from build123d import *

# Parameters (mm, degrees)
SKETCH_1_R          = 2.1
SKETCH_1_R_2        = 6.1
EXTRUDE_1_DEPTH     = 1.5
SKETCH_2_R          = 6.1
SKETCH_2_R_2        = 1.6
CUT_EXTRUDE_1_DEPTH = 53.758885508
FILLET_1_R          = 2


with BuildPart() as part:
    # ｽｹｯﾁ1 → ﾎﾞｽ - 押し出し1 (new body)
    with BuildSketch(Plane.XY):
        with BuildLine():
            ThreePointArc((-37.95979357, -17.309345429), (-38.658047176, -21.61823696), (-35, -24))
            Line((-35, -24), (-14.974979132, -24))
            ThreePointArc((-14.974979132, -24), (0, -35.5), (14.974979132, -24))
            Line((14.974979132, -24), (35, -24))
            ThreePointArc((35, -24), (38.658047176, -21.61823696), (37.95979357, -17.309345429))
            ThreePointArc((37.95979357, -17.309345429), (27.149823207, -3.034907568), (19.058822549, 12.938531129))
            ThreePointArc((19.058822549, 12.938531129), (17.587655142, 14.768604061), (15.342990138, 15.45779162))
            Line((15.342990138, 15.45779162), (-15.342990138, 15.45779162))
            ThreePointArc((-15.342990138, 15.45779162), (-17.587655142, 14.768604061), (-19.058822549, 12.938531129))
            ThreePointArc((-19.058822549, 12.938531129), (-27.149823207, -3.034907568), (-37.95979357, -17.309345429))
        make_face()
        with Locations((-35, -20)):
            Circle(SKETCH_1_R, mode=Mode.SUBTRACT)
        with Locations((0, -20)):
            Circle(SKETCH_1_R_2, mode=Mode.SUBTRACT)
        with Locations((35, -20)):
            Circle(SKETCH_1_R, mode=Mode.SUBTRACT)
        with Locations((-15.342990138, 11.45779162)):
            Circle(SKETCH_1_R, mode=Mode.SUBTRACT)
        with Locations((15.342990138, 11.45779162)):
            Circle(SKETCH_1_R, mode=Mode.SUBTRACT)
    extrude(amount=EXTRUDE_1_DEPTH)

    # ｽｹｯﾁ2 → ｶｯﾄ - 押し出し1 (cut, through all)
    with BuildSketch(Plane.XY.offset(1.5)):
        with Locations((0, -20)):
            Circle(SKETCH_2_R)
        with Locations((23.015, -20)):
            Circle(SKETCH_2_R_2)
        with Locations(Location((-23.015, -20, 0), (0, 0, 180))):
            Circle(SKETCH_2_R_2)
        with Locations((16.215, -20)):
            Circle(SKETCH_2_R_2)
        with Locations(Location((-16.215, -20, 0), (0, 0, 180))):
            Circle(SKETCH_2_R_2)
    extrude(amount=-CUT_EXTRUDE_1_DEPTH, mode=Mode.SUBTRACT)

    # ﾌｨﾚｯﾄ1
    fillet_1_edges = [part.edges().sort_by_distance(p)[0] for p in [
        (-14.974979132, -24, 0.75),
        (14.974979132, -24, 0.75),
    ]]
    fillet(fillet_1_edges, radius=FILLET_1_R)


solid = part.part
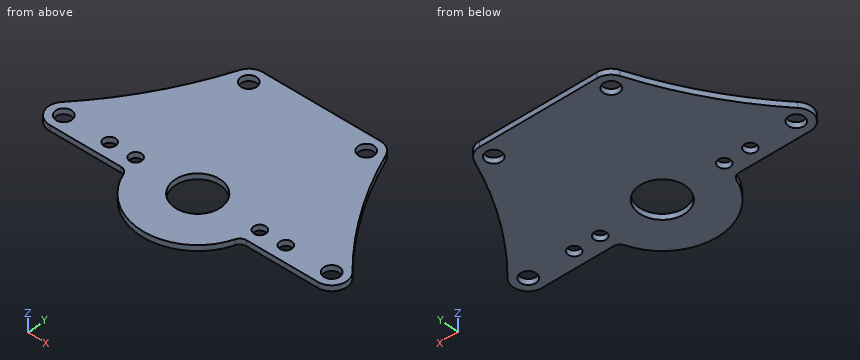
Design review of the part built by this model. Coordinates are the model's own, in mm. Coordinates: 2 decimals unless noted, no trailing zeros. Loops run counter-clockwise (first coordinate to the right, second up) from the corner with the lowest first, then second, coordinate; pieces in that order, holes last.
Item 1: Add section B-B (x = 0). Write out the cut boundary in (y, z), and give its area (3 significant figures).
Completed:
outline: (-35.5, 0) - (-26.1, 0) - (-26.1, 1.5) - (-35.5, 1.5) - close; (-13.9, 0) - (15.46, 0) - (15.46, 1.5) - (-13.9, 1.5) - close
area: 58.1 mm2
Item 2: Add section D-D (x = -12). Write out the cut boundary in (y, z).
Completed:
outline: (-29.81, 0) - (15.46, 0) - (15.46, 1.5) - (-29.81, 1.5) - close
Item 3: Wall thickness on L1, parallel to Y at x = 2, z = 0.8; L2, parallel to Y at x = -1, z = 0.3; L3, parallel to X at y = -3, z = 1.25: over which ranges is each line inside the solid? List them lowest first.
Completed:
L1: y = -35.37 to -25.76, -14.24 to 15.46
L2: y = -35.47 to -26.02, -13.98 to 15.46
L3: x = -27.13 to 27.13
Item 4: Add section A-A (y = -20). Give the number of separate pieces and of enclosed holes in the cut face, and give its area (3 significant figures).
Completed:
separate pieces: 8
enclosed holes: 0
area: 66.9 mm2
Item 5: Clearance check with flat-ended pins moving along their axes: pin 1 (1 mm diameter, centred on x = 1.5, y = -28, fed in from -Z); pin 2 (0.8 mm diameter, centred on x = 28.5, z = 1, fed in from -Y). State where each tip first meets the part, or that it passes through.
Completed:
pin 1: stops at z = 0
pin 2: stops at y = -24
